The model under review builds one solid part; all positions refer to its coordinate system, in mm. Face numbers are marked on the shaded views. A direction names the side the tool comes from. Give positions to 0.01 mm unless a question says otherwise; leave off trailing zeros. Order: outer loops, then holes, each group sorted by start corner. A loop starts at its lowest first (then second) coordinate and runs counter-clockwise, first axis right, second up.
```python
from build123d import *

# Parameters (mm, degrees)
F1_DEPTH = 3
F3_DEPTH = 1
F5_R     = 1.5
F6_DEPTH = 10


with BuildPart() as f1:
    # F0 (on Top) → F1 (new body)
    with BuildSketch(Plane.XY):
        with BuildLine():
            Line((-3.5, 21.073285), (-37, 1.732051))
            ThreePointArc((-37, 1.732051), (-38, 0), (-37, -1.732051))
            Line((-37, -1.732051), (-29.831544, -5.870761))
            ThreePointArc((-29.831544, -5.870761), (-27.245228, -6.748697), (-24.519811, -6.570064))
            Line((-24.519811, -6.570064), (-1.811733, -0.485452))
            ThreePointArc((-1.811733, -0.485452), (0, -0.246933), (1.811733, -0.485452))
            Line((1.811733, -0.485452), (13.088096, -3.506945))
            ThreePointArc((13.088096, -3.506945), (15.191419, -3.299786), (16.636192, -1.757218))
            Line((16.636192, -1.757218), (20.725817, 8.116009))
            ThreePointArc((20.725817, 8.116009), (20.794968, 10.228378), (19.454178, 11.862136))
            Line((19.454178, 11.862136), (3.5, 21.073285))
            ThreePointArc((3.5, 21.073285), (0, 22.011107), (-3.5, 21.073285))
        make_face()
        with BuildLine():
            Line((17.816219, 8.930998), (13.989385, -0.307797))
            ThreePointArc((13.989385, -0.307797), (12.906993, -1.39019), (11.376259, -1.39019))
            Line((11.376259, -1.39019), (-4.791633, 5.30677))
            ThreePointArc((-4.791633, 5.30677), (-5.874025, 6.389163), (-5.874025, 7.919896))
            Line((-5.874025, 7.919896), (-2.047191, 17.158692))
            ThreePointArc((-2.047191, 17.158692), (-0.964799, 18.241084), (0.565935, 18.241084))
            Line((0.565935, 18.241084), (16.733827, 11.544124))
            ThreePointArc((16.733827, 11.544124), (17.816219, 10.461732), (17.816219, 8.930998))
        make_face(mode=Mode.SUBTRACT)
    extrude(amount=F1_DEPTH)

    # F2 (on face) → F3 (join)
    with BuildSketch(Plane.XY.offset(3)):
        with BuildLine():
            Line((1.811733, -0.485452), (13.088096, -3.506945))
            ThreePointArc((13.088096, -3.506945), (15.191419, -3.299786), (16.636192, -1.757218))
            Line((16.636192, -1.757218), (20.725817, 8.116009))
            ThreePointArc((20.725817, 8.116009), (20.794968, 10.228378), (19.454178, 11.862136))
            Line((19.454178, 11.862136), (3.5, 21.073285))
            ThreePointArc((3.5, 21.073285), (0, 22.011107), (-3.5, 21.073285))
            Line((-3.5, 21.073285), (-37, 1.732051))
            ThreePointArc((-37, 1.732051), (-38, 0), (-37, -1.732051))
            Line((-37, -1.732051), (-29.831544, -5.870761))
            ThreePointArc((-29.831544, -5.870761), (-27.245228, -6.748697), (-24.519811, -6.570064))
            Line((-24.519811, -6.570064), (-1.811733, -0.485452))
            ThreePointArc((-1.811733, -0.485452), (0, -0.246933), (1.811733, -0.485452))
        make_face()
        with BuildLine():
            ThreePointArc((-4.447218, 6.138262), (-5.042533, 6.733578), (-5.042533, 7.575481))
            Line((-5.042533, 7.575481), (-1.215699, 16.814277))
            ThreePointArc((-1.215699, 16.814277), (-0.620383, 17.409592), (0.22152, 17.409592))
            Line((0.22152, 17.409592), (16.389412, 10.712632))
            ThreePointArc((16.389412, 10.712632), (16.984728, 10.117316), (16.984728, 9.275413))
            Line((16.984728, 9.275413), (13.157893, 0.036618))
            ThreePointArc((13.157893, 0.036618), (12.562578, -0.558698), (11.720674, -0.558698))
            Line((11.720674, -0.558698), (-4.447218, 6.138262))
        make_face(mode=Mode.SUBTRACT)
    extrude(amount=F3_DEPTH)

    # F5 (on face) → F6 (join)
    with BuildSketch(Plane(origin=(-10, 17.320508, 0), x_dir=(-0.866025, -0.5, 0), z_dir=(-0.5, 0.866025, 0))):
        with BuildLine():
            ThreePointArc((15.611969, -8.308743), (16.033625, -7.188429), (16.176915, -6))
            ThreePointArc((16.176915, -6), (9.988485, -1.14329), (6.74186, -8.308743))
            ThreePointArc((6.74186, -8.308743), (11.176915, -11), (15.611969, -8.308743))
        make_face()
        with Locations((11.176915, -6)):
            Circle(F5_R, mode=Mode.SUBTRACT)
        with BuildLine():
            ThreePointArc((6.74186, -8.308743), (9.988485, -1.14329), (16.176915, -6))
            ThreePointArc((16.176915, -6), (16.033625, -7.188429), (15.611969, -8.308743))
            Line((15.611969, -8.308743), (19.937227, 0))
            Line((19.937227, 0), (2.416602, 0))
            Line((2.416602, 0), (6.74186, -8.308743))
        make_face()
    extrude(amount=-F6_DEPTH)


solid = f1.part
```
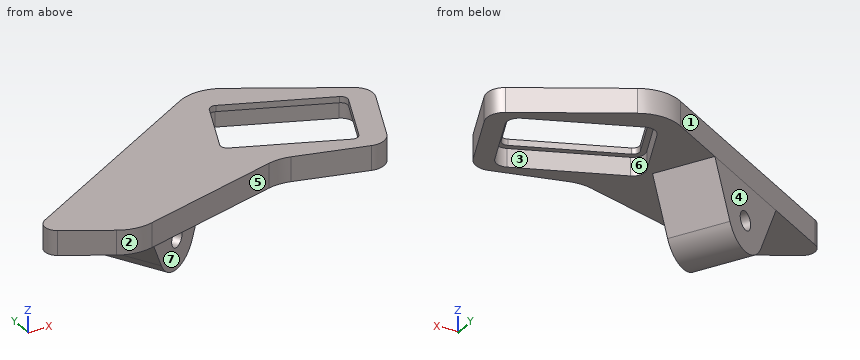
1. Take a section at A-A (z = 1). Write out the cut boundary in (x, y), and give its area (3 significant figures).
2. Draft analysis for pull direction X (two halves, no side actions). For the marked faces 1, 2 and 3, state which applies: pulls with the +X half, pulls with the -X half, needs draft (parallel to the pull), parting line crosses it, or undercut.
3. To check wall thickness, follow line 1 (Z direction, x = -26, y = 0); line 2 (X direction, y = 8.25, z = 1.75); line 3 (X direction, y = 15.5, z = 1.25). State the ranges of each line that lie inside material, in increasing order.
4. Insertion check: pin 1 (4 mm diameter, centred on x = 0.5, y = -2, fed in from -Z); pin 2 (5 mm diameter, centred on y = 14, z = -4.5, fed in from -X); pin 3 (6 mm diameter, centred on y = 15, z = 0, fed in from -X). Each pin has a flat end and moves straight along its axis. Give the tip position at first contact, or say it passes through.
5. For the marked faces 4, 5, 6 and 7, list the 3-axis set-ups (+Z, -Z, +X, -X, +Y, -Y) from which the entire face can be reached by the end or side of a thin tool; tool diameter is ignored.
6. Take a section at B-B (z = -2.25). Write out the cut boundary in (x, y), and give its area (3 significant figures).
7. Take a section at C-C (x = -29). Write out the cut boundary in (y, z).
Answer:
1. outline: (-37, -1.73) - (-29.83, -5.87) arc R7 ccw to (-24.52, -6.57) - (-1.81, -0.49) arc R7 cw to (1.81, -0.49) - (13.09, -3.51) arc R3 ccw to (16.64, -1.76) - (20.73, 8.12) arc R3 ccw to (19.45, 11.86) - (3.5, 21.07) arc R7 ccw to (-3.5, 21.07) - (-37, 1.73) arc R2 ccw to start; hole (-5.87, 7.92) arc R2 ccw to (-4.79, 5.31) - (11.38, -1.39) arc R2 ccw to (13.99, -0.31) - (17.82, 8.93) arc R2 ccw to (16.73, 11.54) - (0.57, 18.24) arc R2 ccw to (-2.05, 17.16) - close
1. area: 681 mm2
2. face 1: pulls with the -X half
2. face 2: parting line crosses it
2. face 3: undercut
3. line 1: z = 0 to 4
3. line 2: x = -25.71 to -5.74, 17.53 to 20.78
3. line 3: x = -13.15 to -2.73, 7.18 to 13.15
4. pin 1: stops at z = 0
4. pin 2: stops at x = -20.08
4. pin 3: stops at x = -19.22
5. face 4: +Z, -Z, -X, +Y
5. face 5: +Z, -Z, -Y
5. face 6: -Z
5. face 7: -Z, +X, -Y
6. outline: (-26.25, 7.94) - (-21.25, -0.72) - (-8.11, 6.87) - (-13.11, 15.53) - close
6. area: 152 mm2
7. outline: (-6.28, 0) - (6.35, 0) - (6.35, 4) - (-6.28, 4) - close
